The drawing under review shows one solid part. Ordinate dimensions are in mm from its lowest x, y, z. Coordinates: 2 decimals unless noted, no trailing zeros. Write each loop counter-clockwise with the first axis right and the second up, starting at its lowest first coordinate (ties: lowest second). Pieces come first, ordered by that corner, then holes. Notation, with made-up numbers: (44, 26) - (61, 26) arc R26 cw to (61, 57) - close; hole circle Ø7 at (-0.75, 79). An arc over 180 degrees is marked (long way). Put each result on its own line as item: value. Start each with the question number.
Item 1: To check wall thickness, follow L1, parallel to Y at x = 49, z = 83; L2, parallel to Z at x = 30, y = 24; L3, parallel to Z at x = 53, y = 8.5. State the ranges of each line that lie inside material, in increasing order. Write a range as [from, to].
Item 2: For pin 1 (2 mm diameter, centred on x = 20, z = 73, fed in from -Y) (1 decimal); pin 2 (5 mm diameter, centred on x = 32.5, z = 84, fed in from +Y); pin 3 (5 mm diameter, centred on x = 14.5, z = 85, fed in from -Y), all flat-tipped, find the tip position at first contact; note any pin that passes through.
Item 3: Consider section C-C on y = 30.5. Give the boundary of the cut face in (x, z).
Item 4: Consider section B-B on y = 25. Give the boundary of the cut face in (x, z) (1 decimal).
Item 5: Consider section A-A on x = 47.5. Give the boundary of the cut face in (y, z) (1 decimal).
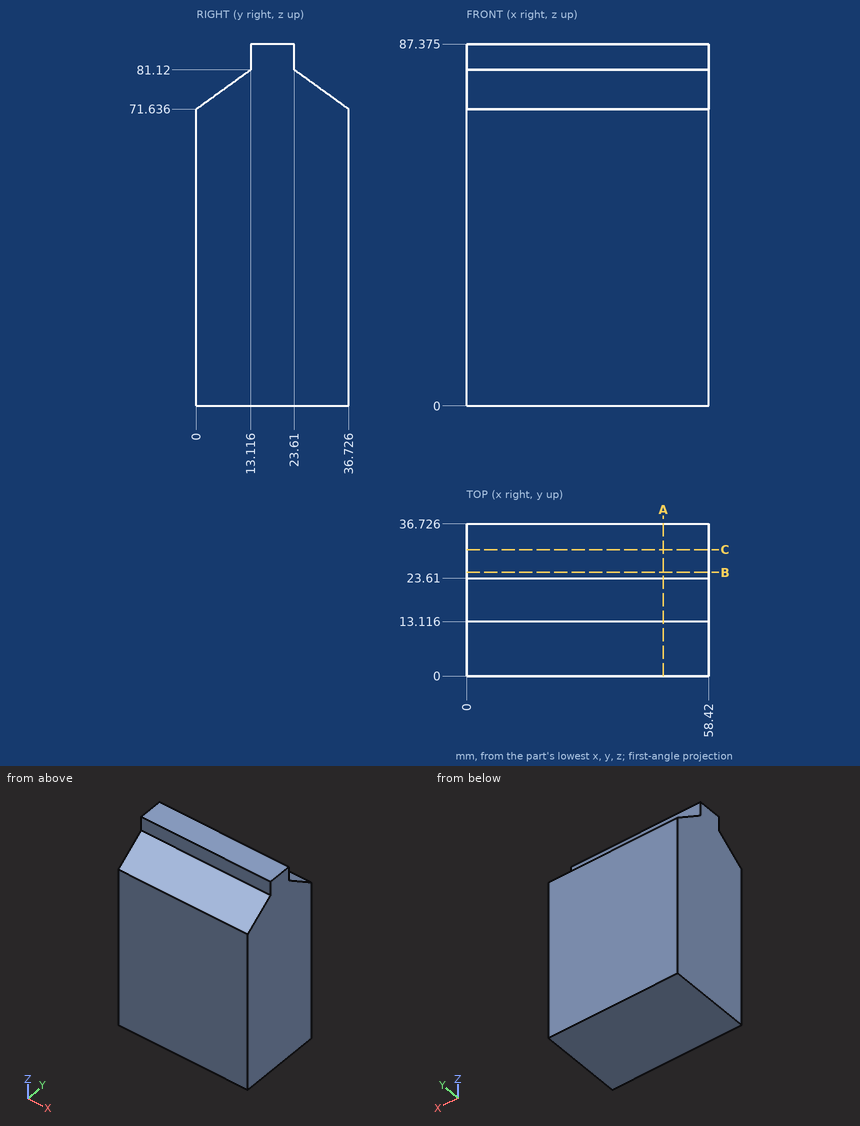
Report:
1. L1: [13.12, 23.61]
1. L2: [0, 80.84]
1. L3: [0, 77.78]
2. pin 1: y = 0.5
2. pin 2: y = 23.61
2. pin 3: y = 13.12
3. outline: (0, 0) - (58.42, 0) - (58.42, 76.14) - (0, 76.14) - close
4. outline: (0, 0) - (58.4, 0) - (58.4, 80.1) - (0, 80.1) - close
5. outline: (0, 0) - (36.7, 0) - (36.7, 71.6) - (23.6, 81.1) - (23.6, 87.4) - (13.1, 87.4) - (13.1, 81.1) - (0, 71.6) - close
